```python
from build123d import *

# Parameters (mm, degrees)
F1_R     = 10.99185
F2_DEPTH = 7
F3_R     = 5.08
F4_R     = 3.49999


# Not quite as in the source:
# - a fillet or chamfer is up to 0.001 mm smaller than in the source, because OpenCascade refuses the exact size


with BuildPart() as f2:
    # F1 (on Top) → F2 (new body)
    with BuildSketch(Plane.XY):
        Polygon((0, 54.0587), (-15.875, 38.1837), (-15.875, -38.1837), (0, -57.15), (15.875, -38.1837), (15.875, 38.1837), align=None)
        with Locations((0, -25.4837)):
            Circle(F1_R, mode=Mode.SUBTRACT)
        Circle(F1_R, mode=Mode.SUBTRACT)
        with Locations((0, 25.4837)):
            Circle(F1_R, mode=Mode.SUBTRACT)
    extrude(amount=F2_DEPTH)

    # F3
    f3_edges = [f2.edges().sort_by_distance(p)[0] for p in [
        (-15.875, -38.1837, 3.5),
        (0, -57.15, 3.5),
        (15.875, -38.1837, 3.5),
        (15.875, 38.1837, 3.5),
        (0, 54.0587, 3.5),
        (-15.875, 38.1837, 3.5),
    ]]
    fillet(f3_edges, radius=F3_R)

    # F4 (radius 3.5 in the source; OpenCascade refuses exactly that, so slightly less here)
    f4_edges = [f2.edges().sort_by_distance(p)[0] for p in [
        (-15.875, -0.129382, 0),
        (15.875, -0.129382, 7),
    ]]
    fillet(f4_edges, radius=F4_R)


solid = f2.part
```
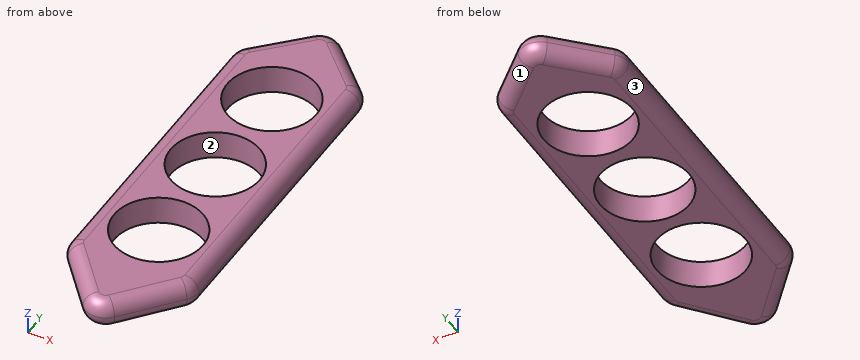
For this review, take the finished solid that the model builds, in its own axes (mm). Face numbers are marked on the shaded views. Coordinates: 2 decimals unless noted, no trailing zeros. Answer in a Markdown table with one row per item. Add a question column.
Q1. Draft analysis for pull direction X (two halves, no side actions). For the marked faces 1, 2 and 3, state which applies: +X half, -X half, draft (parallel to the pull), parting line (faces both ways), or undercut.
Q2. For P1, Ø1.5, axis at y = -10, z = 5, coming from the +X side; P2, Ø3, axis at x = -2, z = 1.5, coming from the +Y side; P3, Ø4, axis at x = 7.5, z = 5.5, coming from the +Y side, all flat-tipped, find the tip position at first contact; note any pin that passes through.
Q3. We need section B-B, the plane x = 0. Count the separate pieces of the cut face and the enclosed holes in it, and give its area (3 significant figures).
Q4. For probe 1 along Y at (x, z) = (-4.5, 2.75); probe 2 along Y at (x, z) = (-3.5, 2.25); probe 3 along X at (y, z) = (2.5, 2.25), list the stretches that pass through material, from the lowest coordinate up.
Answer list:
| question | item | result |
|---|---|---|
| 1 | face 1 | +X half |
| 1 | face 2 | undercut |
| 1 | face 3 | -X half |
| 2 | P1 | stops at x = 15.79 |
| 2 | P2 | stops at y = 51.74 |
| 2 | P3 | stops at y = 48.09 |
| 3 | separate pieces | 4 |
| 3 | enclosed holes | 0 |
| 3 | area | 272 mm2 |
| 4 | probe 1 | y = -51.65 to -35.51, -15.46 to -10.03, 10.03 to 15.46, 35.51 to 49.44 |
| 4 | probe 2 | y = -52.59 to -35.9, -15.06 to -10.42, 10.42 to 15.06, 35.9 to 50.23 |
| 4 | probe 3 | x = -15.64 to -10.7, 10.7 to 15.64 |
